Autodesk Inventor part; units mm, degrees
ref_plane "YZ Plane" through (0, 0, 0) normal (1, 0, 0) x (0, 1, 0)
ref_plane "XZ Plane" through (0, 0, 0) normal (0, 1, 0) x (-1, 0, 0)
ref_plane "XY Plane" through (0, 0, 0) normal (0, 0, 1) x (1, 0, 0)
sketch "Sketch1" plane through (0, 0, 0) normal (0, 0, 1) x (1, 0, 0)
  line L0 (-23.0956, 0) -> (12.4644, 0)
  line L1 (0, -13.335) -> (0, 13.335)
  line L2 (-18.0156, 9.525) -> (-5.3156, 9.525)
  line L3 (7.3844, 0.6324) -> (7.3844, -9.525)
  line L4 (7.3844, -9.525) -> (-18.0156, -9.525)
  line L5 (-18.0156, -9.525) -> (-18.0156, 9.525)
  line L6 (-5.3156, 9.525) -> (7.3844, 0.6324)
  point P0 (0, 0)
  point P1 (-18.0156, 0)
  point P2 (0, 9.525)
  dimension "d0" = 19.05
  dimension "d2" = 25.4
  dimension "d21" = 35
extrude "Extrusion1" add sketch "Sketch1" along normal blind 19.05
sketch "Sketch2" plane through (7.3844, 0.6324, 19.05) normal (0.5736, 0.8192, 0) x (0.8192, -0.5736, 0)
  line L0 (-15.5038, 19.05) -> (0, 19.05)
  line L1 (-15.5038, 19.05) -> (-15.5038, 0)
  point P0 (-5.6862, 19.05)
  point P1 (-7.7519, 9.525)
  point P2 (-15.5038, 9.525)
  point P3 (-7.7519, 19.05)
hole "Hole1" at (1.0344, 5.0787, 9.525) direction (-0.5736, -0.8192, 0) diameter 4.9784 end through all
sketch "Sketch3" plane through (-18.0156, -9.525, 0) normal (0, -1, 0) x (1, 0, 0)
  line L0 (25.4, 0) -> (25.4, 19.05)
  point P0 (18.0156, 0)
  point P1 (19.05, 9.525)
  point P2 (25.4, 9.525)
  point P3 (3.175, 9.525)
  dimension "d12" = 6.35
  dimension "d20" = 15.875
hole "Hole2" at (1.0344, -9.525, 9.525) at (-14.8406, -9.525, 9.525) direction (0, 1, 0) diameter 4.9784 depth 6.35 tip angle 118
properties part number "transfer mount block"
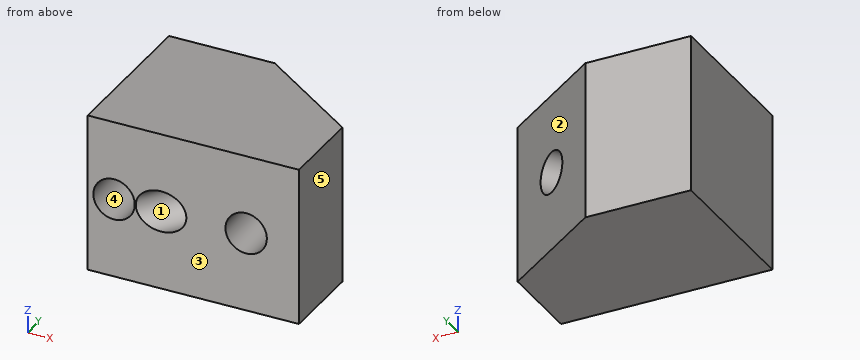
CAD build for the part. Positions are in the model's coordinates, mm. Face numbers are marked on the shaded views. A direction names the side the tool comes from. Round coordinates to 2 decimals unless told otherwise and drop trailing zeros. Order: outer loops, then holes, each group sorted by start corner. A loop starts at its lowest first (then second) coordinate and runs counter-clockwise, first axis right, second up. Notation, with made-up numbers: (27, -22.75) -> (74, -22.75) arc R17 ccw to (74, -14.75) -> close; hole circle Ø5 at (41.25, 25.25). An arc over 180 degrees is marked (long way). Write item = value, one per line.
(1) 3-axis set-ups, long thin cutter, end or side, ignore diameter. For the marked faces 4 and 5: which of +Z, -Z, +X, -X, +Y, -Y reach the whole face in a straight line?
Answers follow:
face_4 = -Y
face_5 = +Z, -Z, +X, +Y, -Y
(2) Cut at A-A (z = 2). Write the cut outline in (x, y) (3 decimals), plus the area to 3 significant figures.
Answers follow:
outline = (-18.016, -9.525) -> (7.384, -9.525) -> (7.384, 0.632) -> (-5.316, 9.525) -> (-18.016, 9.525) -> close
area = 427 mm²
(3) Cut at B-B (y = -2.75). State how many separate pieces and enclosed holes the cut face has, plus the area to 3 significant figures.
Answers follow:
separate_pieces = 1
enclosed_holes = 3
area = 440 mm²
(4) Pull direction Y, two halves, no side cores. Call the marked faces 1, 2 and 3: +Y half, -Y half, draft (parallel to the pull), parting line (faces both ways), or undercut.
Answers follow:
face_1 = undercut
face_2 = +Y half
face_3 = -Y half
(5) Flat gauge pins, fed straight in: P1, Ø6.5, axis at x = 1.03, z = 9.52, coming from the +Y side; P2, Ø2, axis at y = 6.5, z = 11.5, coming from the +X side. Where does each tip first touch, or does it go through?
Answers follow:
P1 = 7.36
P2 = 0.34
(6) Drill centre lines: L1, parallel to Z at x = -15, y = -7.75; L2, parallel to X at y = -3.75, z = 9.5; L3, parallel to Z at x = 0.25, y = -3. Where is each one in solid material? Low to high.
Answers follow:
L1 = 0 to 7.04, 12.01 to 19.05
L2 = -18.02 to -17.33, -12.35 to -8.19, -2.11 to -1.45, 3.52 to 7.38
L3 = 0 to 7.47, 11.58 to 19.05
